Check sheet for the drawn part. Datum: minimum x, y, z corner. Units: mm. A direction names the side the tool comes from. Give positions to 0.01 mm unless a question says otherwise; leave off trailing zeros. Order: outer loops, then holes, each group sorted by start corner. A loop starts at its lowest first (then second) coordinate and runs counter-clockwise, first axis right, second up. Notation, with made-up numbers: M 82.5,61 L 117.5,61 A23 ccw 117.5,95 Z; hole C 14.25,-18 d6. An arc over 180 degrees is marked long. Put each result on its own line as item: value. Start each with the question number.
Q1. Section check A-A on x = 23.9. Record the cut outline in (y, z).
Q2. Access from +Z, -Z, +X, -X, +Y, -Y to the whole of each face (thin tool, end or side, straight path). Record for the marked faces 1 and 2.
Q3. Go/stop test with flat-tipped pins: pin 1 (6 mm diameter, centred on x = 13, y = 22.5, fed in from -Z); pin 2 (2 mm diameter, centred on y = 35.5, z = 13, fed in from -X); pin 3 (1 mm diameter, centred on x = 22.5, z = 43, fed in from +Y). Record where each tip stops, or that it passes through.
Q4. Material ranges on L1, parallel to Y at x = 14, z = 24; L2, parallel to Z at x = 24.5, y = 17; L3, parallel to Z at x = 38.5, y = 37, recorded low to high.
Q5. Section check B-B on y = 27.5. Record the cut outline in (x, z), then the cut area to 3 significant figures.
Q6. Section check C-C on y = 32.5. Record the cut outline in (x, z).
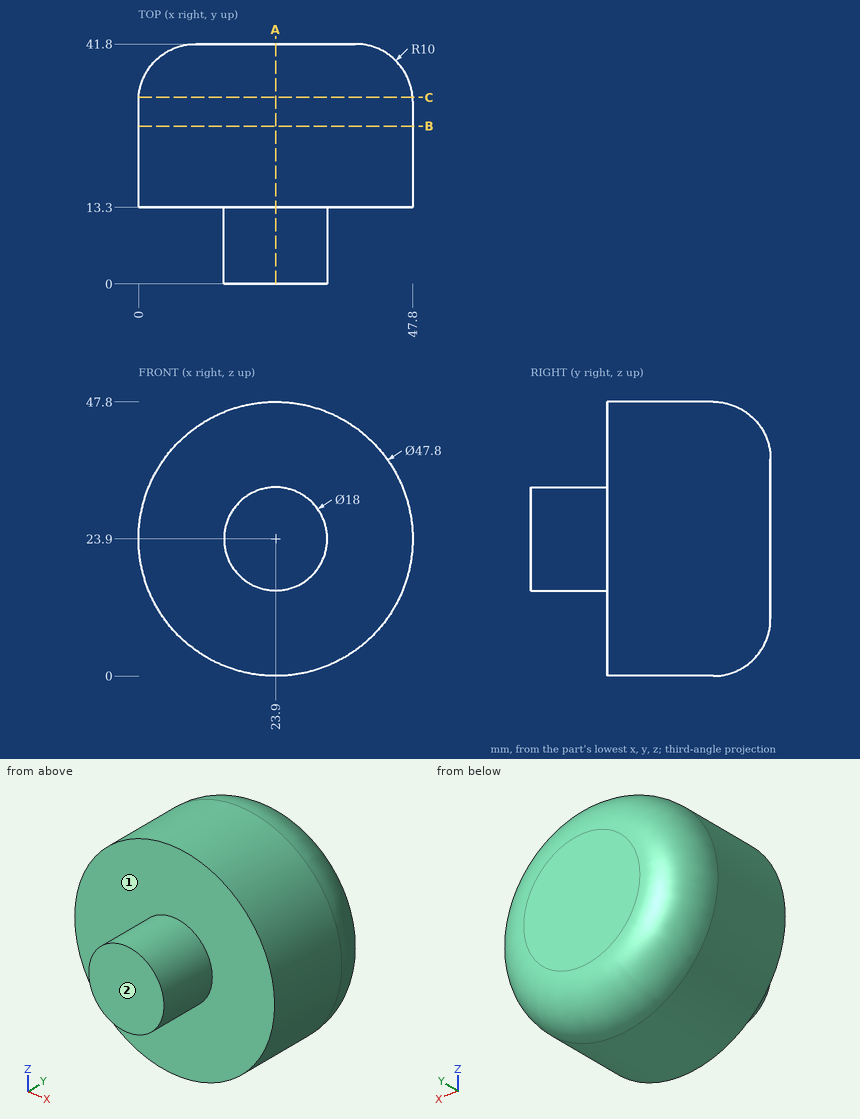
Results found:
1. outline: M 0,14.9 L 13.3,14.9 L 13.3,0 L 31.8,0 A10 ccw 41.8,10 L 41.8,37.8 A10 ccw 31.8,47.8 L 13.3,47.8 L 13.3,32.9 L 0,32.9 Z
2. face 1: -Y
2. face 2: +Z, -Z, +X, -X, -Y
3. pin 1: stops at z = 1.34
3. pin 2: stops at x = 2.78
3. pin 3: stops at y = 40.6
4. L1: y = 13.3 to 41.8
4. L2: z = 0.01 to 47.79
4. L3: z = 6.86 to 40.94
5. outline: C 23.9,23.9 d47.8
5. area: 1,790 mm^2
6. outline: C 23.9,23.9 d47.75
